Source: CAD feature listing. Evaluate the final solid. Frame: model axes, mm. Face numbers are marked on the shaded views. A direction names the side the tool comes from. Give positions to 0.01 mm unless a question says otherwise; leave off trailing zeros. Write each loop counter-clockwise with the first axis right and the second up, starting at its lowest first coordinate (ties: lowest second). Pieces come first, ordered by that corner, then holes. Notation, with made-up numbers: M 71,-22.75 L 79,-22.75 A25 cw 79,-2.75 Z; hole C 53.25,40.25 d5. An arc over 180 degrees is marked long. Use CSV: the item, a comma, the result in double quotes. Start each with the question number.
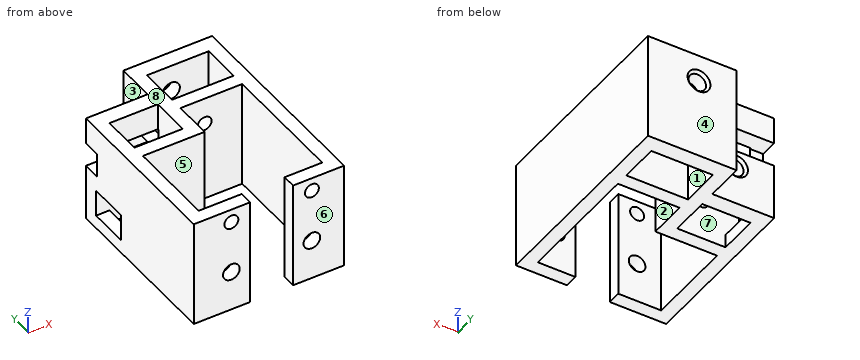
from build123d import *

# Parameters (mm, degrees)
SKETCH1_W           = 23
SKETCH1_H           = 14.75
SKETCH1_W_2         = 18
BOSS_EXTRUDE1_DEPTH = 40
CUT_EXTRUDE1_REACH  = 106.057
SKETCH2_R           = 2.6
CUT_EXTRUDE2_REACH  = 94.064
SKETCH3_W           = 9
SKETCH3_H           = 14.75
SKETCH4_W           = 10
SKETCH4_H           = 14.75
CUT_EXTRUDE3_DEPTH  = 102.453449917
CUT_EXTRUDE4_REACH  = 106.057
SKETCH6_R           = 3.25
CHAMFER1_SIZE       = 1
CUT_EXTRUDE5_REACH  = 106.057
SKETCH7_R           = 2.6
SKETCH7_R_2         = 3.1


with BuildPart() as part:
    # Sketch1 → Boss-Extrude1 (new body)
    with BuildSketch(Plane.XY):
        Polygon((0, 0), (0, 63.75), (23, 63.75), (23, 78.05), (56, 78.05), (56, 0), (37, 0), (37, 5), (51, 5), (51, 52.3), (28, 52.3), (28, 38), (5, 38), (5, 5), (21, 5), (21, 0), align=None)
        with Locations((39.5, 64.675)):
            Rectangle(SKETCH1_W, SKETCH1_H, mode=Mode.SUBTRACT)
        with Locations((14, 50.375)):
            Rectangle(SKETCH1_W_2, SKETCH1_H, mode=Mode.SUBTRACT)
    extrude(amount=BOSS_EXTRUDE1_DEPTH)

    # Cut-Extrude1: up to this face of the body (flat: up to its plane)
    cut_extrude1_end = Plane(part.part.faces().sort_by_distance((16.5, 38, 20))[0])
    # Sketch2 → Cut-Extrude1 (cut, up to the picked face)
    with BuildSketch(Plane(origin=(0, 78.05, 0), x_dir=(1, 0, 0), z_dir=(0, 1, 0)), mode=Mode.PRIVATE) as cut_extrude1_sk1:
        with Locations(Location((14, -15, 0), (0, 0, 270))):
            Circle(SKETCH2_R)
    cut_extrude1_tool1 = split(extrude(cut_extrude1_sk1.sketch, amount=-CUT_EXTRUDE1_REACH, mode=Mode.PRIVATE), bisect_by=cut_extrude1_end, keep=Keep.BOTH, mode=Mode.PRIVATE)
    # Sketch2 → Cut-Extrude1 (cut, up to the picked face)
    with BuildSketch(Plane(origin=(0, 78.05, 0), x_dir=(1, 0, 0), z_dir=(0, 1, 0)), mode=Mode.PRIVATE) as cut_extrude1_sk2:
        with Locations((37, -30)):
            Circle(SKETCH2_R)
    cut_extrude1_tool2 = split(extrude(cut_extrude1_sk2.sketch, amount=-CUT_EXTRUDE1_REACH, mode=Mode.PRIVATE), bisect_by=cut_extrude1_end, keep=Keep.BOTH, mode=Mode.PRIVATE)
    add(cut_extrude1_tool1.solids().sort_by(Axis((14, 78.05, 15), (0, -1, 0)))[0], mode=Mode.SUBTRACT)
    add(cut_extrude1_tool2.solids().sort_by(Axis((37, 78.05, 30), (0, -1, 0)))[0], mode=Mode.SUBTRACT)

    # Sketch3 → Cut-Extrude2 (cut, up to next)
    with BuildSketch(Plane(origin=(28, 0, 0), x_dir=(0, 0, -1), z_dir=(1, 0, 0)), mode=Mode.PRIVATE) as cut_extrude2_sk1:
        with Locations((-25.5, 64.675)):
            Rectangle(SKETCH3_W, SKETCH3_H)
    cut_extrude2_tool1 = extrude(cut_extrude2_sk1.sketch, amount=-CUT_EXTRUDE2_REACH, mode=Mode.PRIVATE) & part.part
    add(cut_extrude2_tool1.solids().sort_by_distance((28, 64.675, 25.5))[0], mode=Mode.SUBTRACT)

    # Sketch4 → Cut-Extrude3 (cut, through all)
    with BuildSketch(Plane(origin=(5, 0, 0), x_dir=(0, 0, -1), z_dir=(1, 0, 0))):
        with Locations((-10, 50.375)):
            Rectangle(SKETCH4_W, SKETCH4_H)
    extrude(amount=-CUT_EXTRUDE3_DEPTH, mode=Mode.SUBTRACT)

    # Sketch6 → Cut-Extrude4 (cut, up to next)
    with BuildSketch(Plane(origin=(0, 78.05, 0), x_dir=(1, 0, 0), z_dir=(0, 1, 0)), mode=Mode.PRIVATE) as cut_extrude4_sk1:
        with Locations(Location((14, -15, 0), (0, 0, 270))):
            Circle(SKETCH6_R)
    cut_extrude4_tool1 = extrude(cut_extrude4_sk1.sketch, amount=-CUT_EXTRUDE4_REACH, mode=Mode.PRIVATE) & part.part
    # Sketch6 → Cut-Extrude4 (cut, up to next)
    with BuildSketch(Plane(origin=(0, 78.05, 0), x_dir=(1, 0, 0), z_dir=(0, 1, 0)), mode=Mode.PRIVATE) as cut_extrude4_sk2:
        with Locations(Location((37, -30, 0), (0, 0, 270))):
            Circle(SKETCH6_R)
    cut_extrude4_tool2 = extrude(cut_extrude4_sk2.sketch, amount=-CUT_EXTRUDE4_REACH, mode=Mode.PRIVATE) & part.part
    add(cut_extrude4_tool1.solids().sort_by_distance((14, 78.05, 15))[0], mode=Mode.SUBTRACT)
    add(cut_extrude4_tool2.solids().sort_by_distance((37, 78.05, 30))[0], mode=Mode.SUBTRACT)

    # Chamfer1
    chamfer1_edges = [part.edges().sort_by_distance(p)[0] for p in [
        (14, 63.75, 11.75),
        (37, 78.05, 26.75),
    ]]
    chamfer(chamfer1_edges, length=CHAMFER1_SIZE)

    # Sketch7 → Cut-Extrude5 (cut, up to next)
    with BuildSketch(Plane.XZ, mode=Mode.PRIVATE) as cut_extrude5_sk1:
        with Locations((14, 35)):
            Circle(SKETCH7_R)
    cut_extrude5_tool1 = extrude(cut_extrude5_sk1.sketch, amount=-CUT_EXTRUDE5_REACH, mode=Mode.PRIVATE) & part.part
    # Sketch7 → Cut-Extrude5 (cut, up to next)
    with BuildSketch(Plane.XZ, mode=Mode.PRIVATE) as cut_extrude5_sk2:
        with Locations((44, 35)):
            Circle(SKETCH7_R)
    cut_extrude5_tool2 = extrude(cut_extrude5_sk2.sketch, amount=-CUT_EXTRUDE5_REACH, mode=Mode.PRIVATE) & part.part
    # Sketch7 → Cut-Extrude5 (cut, up to next)
    with BuildSketch(Plane.XZ, mode=Mode.PRIVATE) as cut_extrude5_sk3:
        with Locations((14, 15)):
            Circle(SKETCH7_R_2)
    cut_extrude5_tool3 = extrude(cut_extrude5_sk3.sketch, amount=-CUT_EXTRUDE5_REACH, mode=Mode.PRIVATE) & part.part
    # Sketch7 → Cut-Extrude5 (cut, up to next)
    with BuildSketch(Plane.XZ, mode=Mode.PRIVATE) as cut_extrude5_sk4:
        with Locations((44, 15)):
            Circle(SKETCH7_R_2)
    cut_extrude5_tool4 = extrude(cut_extrude5_sk4.sketch, amount=-CUT_EXTRUDE5_REACH, mode=Mode.PRIVATE) & part.part
    add(cut_extrude5_tool1.solids().sort_by_distance((14, 0, 35))[0], mode=Mode.SUBTRACT)
    add(cut_extrude5_tool2.solids().sort_by_distance((44, 0, 35))[0], mode=Mode.SUBTRACT)
    add(cut_extrude5_tool3.solids().sort_by_distance((14, 0, 15))[0], mode=Mode.SUBTRACT)
    add(cut_extrude5_tool4.solids().sort_by_distance((44, 0, 15))[0], mode=Mode.SUBTRACT)


solid = part.part
1. First-contact query: pin 1 (7 mm diameter, centred on x = 11, z = 23, fed in from +Y); pin 2 (3.5 mm diameter, centred on x = 44, z = 15, fed in from -Y); pin 3 (7 mm diameter, centred on y = 70.5, z = 25.5, fed in from -X). Flat tips, straight axial feed; report the tip coordinate or a pass-through.
2. Pull-direction query (Y, two-part tool) for the marked faces 5, 6, 7 and 8; classes: released by +Y, released by -Y, zero draft, split by the parting line, or undercut.
3. Section C-C on x = 14. Give the number of separate pieces and of enclosed holes in the cut face, then the cut area to 3 significant figures.
4. Section D-D on z = 8.5. Return loops of the section in (x, y), then the cut area to 3 significant figures.
5. Section A-A on y = 28.5. Return loops of the section in (x, z), then the cut area to 3 significant figures.
6. Line query: probe 1 along Z at (x, y) = (44, 3); probe 2 along X at (y, z) = (50.5, 3); probe 3 along Y at (x, z) = (49.5, 3). Output: solid intervals per line, ascending.
7. Access query for the marked faces 1, 2, 3 and 4. Directions: +Z, -Z, +X, -X, +Y, -Y. A direction counts if a zero-diameter tool reaches every point of the face in a straight line with its end or side. Return the directions, or none.
8. Section B-B on x = 24.5. Return loops of the section in (y, z), then the cut area to 3 significant figures.
Resolved:
1,pin 1,"stops at y = 63.75"
1,pin 2,"stops at y = 52.3"
1,pin 3,"stops at x = 23"
2,face 5,"undercut"
2,face 6,"released by -Y"
2,face 7,"undercut"
2,face 8,"zero draft"
3,separate pieces,"8"
3,enclosed holes,"0"
3,area,"463 mm2"
4,outline,"M 0,0 L 21,0 L 21,5 L 5,5 L 5,38 L 28,38 L 28,52.3 L 51,52.3 L 51,5 L 37,5 L 37,0 L 56,0 L 56,78.05 L 23,78.05 L 23,63.75 L 0,63.75 L 0,57.75 L 23,57.75 L 23,43 L 0,43 Z; hole M 28,57.3 L 51,57.3 L 51,72.05 L 28,72.05 Z"
4,area,"1,440 mm2"
5,outline,"M 0,0 L 5,0 L 5,40 L 0,40 Z; M 51,0 L 56,0 L 56,40 L 51,40 Z"
5,area,"400 mm2"
6,probe 1,"z = 0 to 11.9, 18.1 to 32.4, 37.6 to 40"
6,probe 2,"x = 0 to 5, 23 to 28, 51 to 56"
6,probe 3,"y = 0 to 5, 52.3 to 57.3, 72.05 to 78.05"
7,face 1,"+Z, -Z"
7,face 2,"+Z, -Z, -Y"
7,face 3,"+Z, -Z, -X, +Y"
7,face 4,"+Z, -Z, +X, -X, +Y"
8,outline,"M 38,0 L 78.05,0 L 78.05,40 L 38,40 Z; hole M 57.3,21 L 72.05,21 L 72.05,30 L 57.3,30 Z"
8,area,"1,470 mm2"
